Input: part model. Units: mm. Frame: model coordinates. Give positions to 0.01 mm unless a question says otherwise; leave off trailing zeros. Order: outer loops, then holes, each group sorted by start corner. A loop starts at its lowest first (then second) coordinate and runs counter-clockwise, first axis right, second up. Notation, with made-up numbers: M 52.5,45 L 78.5,45 A28 cw 78.5,73 Z; hole C 38,20.5 d5. An arc over 180 degrees is marked long. Use a Markdown table: item, result.
Autodesk Inventor part; units mm, degrees
ref_plane "Startebene" through (0, 0, 0) normal (1, 0, 0) x (0, 1, 0)
ref_plane "XZ Plane" through (0, 0, 0) normal (0, 1, 0) x (-1, 0, 0)
ref_plane "XY Plane" through (0, 0, 0) normal (0, 0, 1) x (1, 0, 0)
sketch "Hauptskizze" plane through (0, 0, 0) normal (0, 0, 1) x (1, 0, 0)
  line L0 (0, 0) -> (40, 0)
  line L1 (0, 0) -> (0, 2)
  line L2 (0, 2) -> (31, 2)
  line L3 (40, 2) -> (40, 0)
  line L4 (31, 2) -> (40, 2)
  dimension "d3" = 4
  dimension "d5" = 4
revolve "Umdrehung1" add sketch "Hauptskizze" angle 360 about axis through (0, 0, 0) along (1, 0, 0)
chamfer "Fase1" distance 0.5 angle 45 1 edges at (0, -2, 0) measured on face at (10.3333, 1.9935, -0.1609)
chamfer "Fase2" distance 0.5 angle 45 1 edges at (40, -2, 0) measured on face at (34, 1.9935, -0.1609)
properties part number "Welle" material "Steel"
1) First-contact query: pin 1 Ø2 at (x, z) = (15.5, 1.5) entering from +Y; pin 2 Ø1.5 at (x, y) = (16, -1) entering from +Z. Flat tips, straight axial feed; report the tip coordinate or a pass-through.
Response values:
| item | result |
|---|---|
| pin 1 | stops at y = 1.94 |
| pin 2 | stops at z = 1.98 |
2) Cut plane A-A on x = 27.5. Return loops of the section in (y, z), and give its area (3 significant figures).
Response values:
| item | result |
|---|---|
| outline | C 0,0 d4 |
| area | 12.6 mm² |
3) Material intervals for line 1 (Y direction, x = 4, z = -1.2); line 2 (X direction, y = -1.2, z = -1.05); line 3 (Y direction, x = 25, z = 0.7), sorted ascending. Write a range as from..to.
Response values:
| item | result |
|---|---|
| line 1 | y = -1.6..1.6 |
| line 2 | x = 0.09..39.91 |
| line 3 | y = -1.87..1.87 |
